```python
from build123d import *

# Parameters (mm, degrees)
SKETCH1_R           = 0.95
BOSS_EXTRUDE1_DEPTH = 2


with BuildPart() as part:
    # Sketch1 → Boss-Extrude1 (new body)
    with BuildSketch(Plane.XY):
        with BuildLine():
            Line((0, 22.14), (0, 7))
            Line((0, 7), (4, 7))
            Line((4, 7), (4, 5))
            Line((4, 5), (0, 5))
            Line((0, 5), (0, 2))
            ThreePointArc((0, 2), (0.585786438, 0.585786438), (2, 0))
            Line((2, 0), (14.2, 0))
            ThreePointArc((14.2, 0), (15.614213562, 0.585786438), (16.2, 2))
            Line((16.2, 2), (16.2, 5))
            Line((16.2, 5), (12.2, 5))
            Line((12.2, 5), (12.2, 7))
            Line((12.2, 7), (16.2, 7))
            Line((16.2, 7), (16.2, 22.14))
            Line((16.2, 22.14), (12.2, 22.14))
            Line((12.2, 22.14), (12.2, 24.14))
            Line((12.2, 24.14), (16.2, 24.14))
            Line((16.2, 24.14), (16.2, 27.14))
            ThreePointArc((16.2, 27.14), (15.614213562, 28.554213562), (14.2, 29.14))
            Line((14.2, 29.14), (2, 29.14))
            ThreePointArc((2, 29.14), (0.585786438, 28.554213562), (0, 27.14))
            Line((0, 27.14), (0, 24.14))
            Line((0, 24.14), (4, 24.14))
            Line((4, 24.14), (4, 22.14))
            Line((4, 22.14), (0, 22.14))
        make_face()
        with Locations((13.45, 2.5)):
            Circle(SKETCH1_R, mode=Mode.SUBTRACT)
        with Locations((10.2, 9.5)):
            Circle(SKETCH1_R, mode=Mode.SUBTRACT)
        with Locations((2.75, 26.64)):
            Circle(SKETCH1_R, mode=Mode.SUBTRACT)
        with Locations((6, 19.64)):
            Circle(SKETCH1_R, mode=Mode.SUBTRACT)
        with Locations((6, 9.5)):
            Circle(SKETCH1_R, mode=Mode.SUBTRACT)
        with Locations((2.75, 2.5)):
            Circle(SKETCH1_R, mode=Mode.SUBTRACT)
        with Locations((10.2, 19.64)):
            Circle(SKETCH1_R, mode=Mode.SUBTRACT)
        with Locations((13.45, 26.64)):
            Circle(SKETCH1_R, mode=Mode.SUBTRACT)
    extrude(amount=BOSS_EXTRUDE1_DEPTH)


solid = part.part
```
Could you check a few things on this model? Use its own coordinates, in mm. A direction names the side the tool comes from. Round coordinates to 2 decimals unless told otherwise and drop trailing zeros. Write each loop counter-clockwise with the first axis right and the second up, starting at its lowest first coordinate (ties: lowest second). Pieces come first, ordered by that corner, then holes.
(1) Suppose I cut it at D-D on z = 1.1. State how many separate pieces and enclosed holes the cut face has, and give its area (3 significant figures).
Findings below:
separate pieces: 1
enclosed holes: 8
area: 414 mm2
(2) For pin 1 (1 mm diameter, centred on x = 15, z = 1.5, fed in from +Y); pin 2 (1 mm diameter, centred on y = 6, z = 0.5, fed in from -X), each with a flat end and sliding along its axis, tell me the tip position at first contact or that it passes through.
Findings below:
pin 1: stops at y = 29.12
pin 2: stops at x = 4
(3) Suppose I cut it at B-B on y = 19.64. Write out the boundary of the cut face in (x, z).
Findings below:
outline: (0, 0) - (5.05, 0) - (5.05, 2) - (0, 2) - close; (6.95, 0) - (9.25, 0) - (9.25, 2) - (6.95, 2) - close; (11.15, 0) - (16.2, 0) - (16.2, 2) - (11.15, 2) - close
(4) Which directions (+Z, -Z, +X, -X, +Y, -Y) give clear straight access to the entire face, cutting with the end or side of a thin tool? Please do faces 1 (the face through (12.2, 6, 1)), 2 (the face through (13.96, 27.44, 0.99)), 3 (the face through (4, 6, 1)).
Findings below:
face 1: +Z, -Z, +X
face 2: +Z, -Z
face 3: +Z, -Z, -X
(5) Suppose I cut it at A-A on x = 2.75. Write out the boundary of the cut face in (y, z), and give its area (3 significant figures).
Findings below:
outline: (0, 0) - (1.55, 0) - (1.55, 2) - (0, 2) - close; (3.45, 0) - (5, 0) - (5, 2) - (3.45, 2) - close; (7, 0) - (22.14, 0) - (22.14, 2) - (7, 2) - close; (24.14, 0) - (25.69, 0) - (25.69, 2) - (24.14, 2) - close; (27.59, 0) - (29.14, 0) - (29.14, 2) - (27.59, 2) - close
area: 42.7 mm2
(6) If I drill on probe 1 along X at (y, z) = (19.75, 1.2); probe 2 along Y at (x, z) = (13.45, 1.5); probe 3 along Y at (x, z) = (15.75, 0.5), over which ranges is the centre line in solid material (lowest first)?
Findings below:
probe 1: x = 0 to 5.06, 6.94 to 9.26, 11.14 to 16.2
probe 2: y = 0 to 1.55, 3.45 to 5, 7 to 22.14, 24.14 to 25.69, 27.59 to 29.14
probe 3: y = 0.74 to 5, 7 to 22.14, 24.14 to 28.4
(7) Suppose I cut it at C-C on x = 6. Write out the boundary of the cut face in (y, z), and give its area (3 significant figures).
Findings below:
outline: (0, 0) - (8.55, 0) - (8.55, 2) - (0, 2) - close; (10.45, 0) - (18.69, 0) - (18.69, 2) - (10.45, 2) - close; (20.59, 0) - (29.14, 0) - (29.14, 2) - (20.59, 2) - close
area: 50.7 mm2
